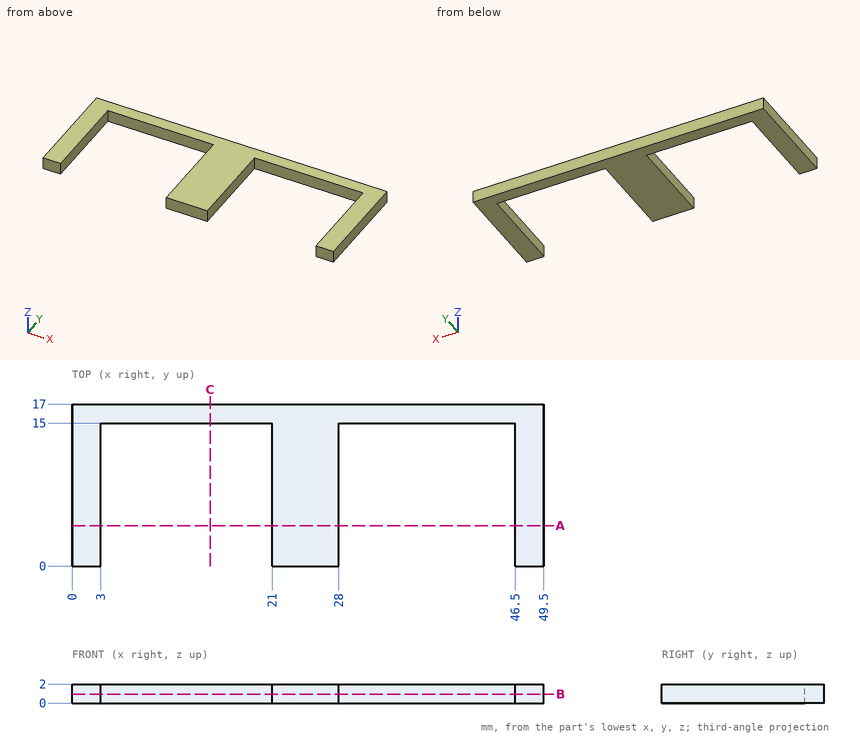
Input: dimensioned drawing with shaded views. Units: mm. Origin: part minimum x, y, z. Give positions to 0.01 mm unless a question says otherwise; leave off trailing zeros. Order: outer loops, then holes, each group sorted by start corner. A loop starts at its lowest first (then second) coordinate and runs counter-clockwise, first axis right, second up. Notation, with made-up numbers: (61, -39) -> (74, -39) arc R22 cw to (74, -6) -> close; hole circle Ø7 at (59, 55). An arc over 180 degrees is marked (long way). Answer as a JSON object with one key per item and string values.
Q1. Section B-B (z = 0.95). Output: boundary loops of the cut face in (x, y), plus the area to 3 significant figures.
Entries:
{"outline": "(0, 0) -> (3, 0) -> (3, 15) -> (21, 15) -> (21, 0) -> (28, 0) -> (28, 15) -> (46.5, 15) -> (46.5, 0) -> (49.5, 0) -> (49.5, 17) -> (0, 17) -> close", "area": "294 mm^2"}
Q2. Material intervals for probe 1 along X at (y, z) = (14.75, 0.7); probe 2 along Y at (x, z) = (44, 0.2), sorted ascending.
Entries:
{"probe 1": "x = 0 to 3, 21 to 28, 46.5 to 49.5", "probe 2": "y = 15 to 17"}
Q3. Section C-C (x = 14.5). Output: boundary loops of the cut face in (y, z), plus the area to 3 significant figures.
Entries:
{"outline": "(15, 0) -> (17, 0) -> (17, 2) -> (15, 2) -> close", "area": "4.00 mm^2"}
Q4. Section A-A (y = 4.25). Output: boundary loops of the cut face in (x, z), plus the area to 3 significant figures.
Entries:
{"outline": "(0, 0) -> (3, 0) -> (3, 2) -> (0, 2) -> close; (21, 0) -> (28, 0) -> (28, 2) -> (21, 2) -> close; (46.5, 0) -> (49.5, 0) -> (49.5, 2) -> (46.5, 2) -> close", "area": "26.0 mm^2"}
